Autodesk Fusion 360 part; units mm, degrees
sketch "Sketch1" plane through (0, 0, 0) normal (0, 0, 1) x (1, 0, 0)
  line L0 (0, 0) -> (46, 0)
  line L1 (46, 0) -> (46, 80)
  line L2 (46, 80) -> (0, 80)
  line L3 (0, 80) -> (0, 0)
  dimension "d1" = 46
  dimension "d2" = 80
extrude "Extrude1" add sketch "Sketch1" along normal blind 20
shell "Shell1" thickness 2 removed faces 1 at (15.3333, 53.3333, 20)
sketch "Sketch2" plane through (0, 0, 0) normal (0, -1, 0) x (1, 0, 0)
  line L0 (0, 0) -> (46, 0)
  line L1 (46, 0) -> (46, 20)
  line L2 (46, 20) -> (0, 20)
  line L3 (0, 20) -> (0, 0)
  line L4 (46, 20) -> (41, 20)
  line L5 (41, 20) -> (41, -16.068)
  line L6 (41, -16.068) -> (46, -16.068)
  line L7 (46, -16.068) -> (46, 20)
  line L8 (0, 0) -> (5, 0)
  line L9 (5, 0) -> (5, 36.068)
  line L10 (5, 36.068) -> (0, 36.068)
  line L11 (0, 36.068) -> (0, 0)
  line L12 (46, 0) -> (0, 0)
  line L13 (0, 0) -> (0, 2)
  line L14 (0, 2) -> (46, 2)
  line L15 (46, 2) -> (46, 0)
  dimension "d6" = 5
  dimension "d7" = 5
  dimension "d8" = 2
extrude "Extrude2" cut sketch "Sketch2" against normal blind 155 contours L2 L5 L9 L14
sketch "Sketch3" plane through (46, 0, 0) normal (1, 0, 0) x (0, 1, 0)
  line L0 (0, 0) -> (80, 0)
  line L1 (80, 0) -> (80, 20)
  line L2 (80, 20) -> (0, 20)
  line L3 (0, 20) -> (0, 0)
  line L4 (80, 0) -> (56, 0)
  line L5 (56, 0) -> (56, 36.068)
  line L6 (56, 36.068) -> (80, 36.068)
  line L7 (80, 36.068) -> (80, 0)
  line L8 (0, 20) -> (24, 20)
  line L9 (24, 20) -> (24, -16.068)
  line L10 (24, -16.068) -> (0, -16.068)
  line L11 (0, -16.068) -> (0, 20)
  line L12 (0, 0) -> (142, 0)
  line L13 (142, 0) -> (142, 2)
  line L14 (142, 2) -> (0, 2)
  line L15 (0, 2) -> (0, 0)
  dimension "d11" = 24
  dimension "d12" = 24
  dimension "d13" = 2
extrude "Extrude3" cut sketch "Sketch3" against normal blind 15 contours L2 L5 L9 L14
Work out the finished part from the listing and answer in its coordinate system (mm). A direction names the side the tool comes from. Round coordinates to 2 decimals unless told otherwise and drop trailing zeros. Order: outer loops, then holes, each group sorted by start corner. A loop starts at its lowest first (then second) coordinate and runs counter-clockwise, first axis right, second up. Notation, with made-up numbers: M 65.5,54 L 81.5,54 A27 cw 81.5,85 Z; hole C 87,56.5 d9. An arc over 180 degrees is marked long. Put each result on its own line as item: value. Start each with the question number.
Q1. For a pull along X with two mould halves and no side action, classify faces 4 (the flat face through (0, 41, 10)), 5 (the flat face through (41, 79, 11)), 6 (the flat face through (21.2, 0, 1.8)) as pulls with the +X half, pulls with the -X half, needs draft (parallel to the pull), parting line crosses it, or undercut.
Q2. Section D-D, the plane y = 42.5 is taken. Write down the section's boundary in (x, z).
Q3. A flat-ended cylindrical pin translates along its axis: pin 1 (10 mm diameter, centred on x = 17, y = 67, fed in from +Z). Find the tip coordinate at first contact, or state that the pin passes through.
Q4. Section A-A, the plane z = 3.25 is taken. Write down the section's boundary in (x, y), and give its area (3 significant figures).
Q5. A tool of negligible diameter and unlimited length cuts with its end or side. For faces 1 (the flat face through (5, 79, 11)), 2 (the flat face through (45, 24, 11)), 3 (the flat face through (44, 13, 11)), from which of +Z, -Z, +X, -X, +Y, -Y can it reach the whole face along a straight path? Write none if from no direction.
Q6. Section B-B, the plane y = 9.5 is taken. Write down the section's boundary in (x, z).
Q7. Straight lines are drawn through the part: L1, parallel to X at y = 3, z = 6.75; L2, parallel to Y at x = 41.5, z = 4.75; L3, parallel to Z at x = 30, y = 62.5. For each, find the intervals that lie inside material, in ascending order. Write a range as [from, to].
Q8. Section C-C, the plane x = 13.5 is taken. Write down the section's boundary in (y, z), and give its area (3 significant figures).
Findings below:
1. face 4: pulls with the -X half
1. face 5: undercut
1. face 6: needs draft
2. outline: M 0,0 L 46,0 L 46,2 L 2,2 L 2,20 L 0,20 Z
3. pin 1: stops at z = 2
4. outline: M 0,0 L 5,0 L 5,2 L 2,2 L 2,78 L 5,78 L 5,80 L 0,80 Z; M 41,0 L 46,0 L 46,24 L 44,24 L 44,2 L 41,2 Z; M 41,78 L 44,78 L 44,56 L 46,56 L 46,80 L 41,80 Z
4. area: 280 mm^2
5. face 1: +Z, +Y, -Y
5. face 2: +Z, +X
5. face 3: +Z
6. outline: M 0,0 L 46,0 L 46,20 L 44,20 L 44,2 L 2,2 L 2,20 L 0,20 Z
7. L1: x = [0, 2], [44, 46]
7. L2: y = [0, 2], [78, 80]
7. L3: z = [0, 2]
8. outline: M 0,0 L 80,0 L 80,2 L 0,2 Z
8. area: 160 mm^2
